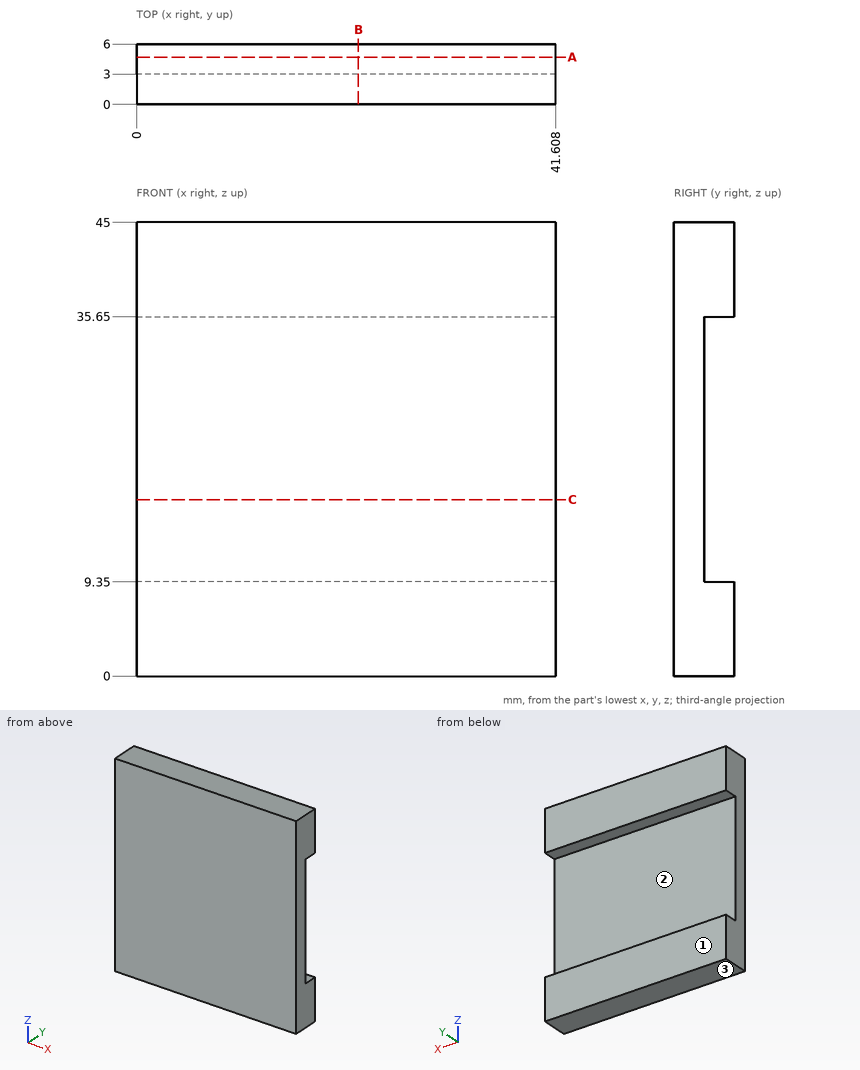
Check sheet for the drawn part. Datum: minimum x, y, z corner. Units: mm. Give positions to 0.01 mm unless a question says otherwise; leave off trailing zeros. Order: outer loops, then holes, each group sorted by start corner. A loop starts at its lowest first (then second) coordinate and runs counter-clockwise, first axis right, second up. Notation, with made-up numbers: (-30, 74.5) - (24, 74.5) arc R20 cw to (24, 98.5) - close; hole circle Ø10 at (31, 33.25). An arc over 180 degrees is marked (long way). Write item = value, one per line. Start each with the question number.
1) Gauge pin test, flat end, axial feed: pin 1 Ø21 at (x, z) = (26, 22.5) entering from +Y. Record the tip position at first contact, or that the pin passes through.
2) Section check C-C (z = 17.5). Enter the section's corners in (x, y).
3) Section check B-B (x = 22). Enter the section's corners in (y, z), then the cut area to 3 significant figures.
4) Section check A-A (y = 4.7). Enter the section's corners in (x, z).
5) Scan lines: L1, parallel to Z at x = 11, y = 5.3; L2, parallel to Y at x = 28, z = 33.5. Record each from-to range of solid material in increasing order.
6) Draft check along Z on the marked faces 1, 2 and 3. Enter one of: released by +Z, released by -Z, zero draft, split by the parting line, or undercut.
Geometry check:
q1.pin_1 = 3
q2.outline = (0, 0) - (41.61, 0) - (41.61, 3) - (0, 3) - close
q3.outline = (0, 0) - (6, 0) - (6, 9.35) - (3, 9.35) - (3, 35.65) - (6, 35.65) - (6, 45) - (0, 45) - close
q3.area = 191 mm2
q4.outline = (0, 0) - (41.61, 0) - (41.61, 9.35) - (0, 9.35) - close; (0, 35.65) - (41.61, 35.65) - (41.61, 45) - (0, 45) - close
q5.L1 = 0 to 9.35, 35.65 to 45
q5.L2 = 0 to 3
q6.face_1 = zero draft
q6.face_2 = undercut
q6.face_3 = released by -Z
